```python
from build123d import *

# Parameters (mm, degrees)
F0_R     = 3
F1_DEPTH = 3
F3_DEPTH = 11.5
F4_R     = 0.5
F6_DEPTH = 3.5
F7_D     = 3


with BuildPart() as f1:
    # F0 (on Top) → F1 (new body)
    with BuildSketch(Plane.XY):
        with BuildLine():
            ThreePointArc((-53.0873338103, 3.9548860426), (-48.0828963467, 9.2999784643), (-46.2654588103, 16.393026337))
            ThreePointArc((-46.2654588103, 16.393026337), (-48.0828963467, 23.4860742098), (-53.0873338103, 28.8311666315))
            ThreePointArc((-53.0873338103, 28.8311666315), (-61.0154588103, 31.143026337), (-68.9435838103, 28.8311666315))
            ThreePointArc((-68.9435838103, 28.8311666315), (-75.7654588103, 16.393026337), (-68.9435838103, 3.9548860426))
            ThreePointArc((-68.9435838103, 3.9548860426), (-61.0154588103, 1.643026337), (-53.0873338103, 3.9548860426))
        make_face()
        with BuildLine():
            ThreePointArc((-68.9435838103, 3.9548860426), (-75.7654588103, 16.393026337), (-68.9435838103, 28.8311666315))
            Line((-68.9435838103, 28.8311666315), (-83.1654588103, 19.7660813321))
            ThreePointArc((-83.1654588103, 19.7660813321), (-79.0919204042, 19.9001619204), (-77.0154588103, 16.393026337))
            ThreePointArc((-77.0154588103, 16.393026337), (-79.0919204042, 12.8858907537), (-83.1654588103, 13.0199713419))
            Line((-83.1654588103, 13.0199713419), (-68.9435838103, 3.9548860426))
        make_face()
        with BuildLine():
            ThreePointArc((-53.0873338103, 28.8311666315), (-48.0828963467, 23.4860742098), (-46.2654588103, 16.393026337))
            ThreePointArc((-46.2654588103, 16.393026337), (-48.0828963467, 9.2999784643), (-53.0873338103, 3.9548860426))
            Line((-53.0873338103, 3.9548860426), (-38.8654588103, 13.0199713419))
            ThreePointArc((-38.8654588103, 13.0199713419), (-45.0154588103, 16.393026337), (-38.8654588103, 19.7660813321))
            Line((-38.8654588103, 19.7660813321), (-53.0873338103, 28.8311666315))
        make_face()
        with BuildLine():
            ThreePointArc((-37.0154588103, 16.393026337), (-37.508323227, 18.3165647432), (-38.8654588103, 19.7660813321))
            ThreePointArc((-38.8654588103, 19.7660813321), (-45.0154588103, 16.393026337), (-38.8654588103, 13.0199713419))
            ThreePointArc((-38.8654588103, 13.0199713419), (-37.508323227, 14.4694879309), (-37.0154588103, 16.393026337))
        make_face()
        with Locations((-41.0154588103, 16.393026337)):
            Circle(F0_R, mode=Mode.SUBTRACT)
        with BuildLine():
            ThreePointArc((-77.0154588103, 16.393026337), (-79.0919204042, 19.9001619204), (-83.1654588103, 19.7660813321))
            ThreePointArc((-83.1654588103, 19.7660813321), (-85.0154588103, 16.393026337), (-83.1654588103, 13.0199713419))
            ThreePointArc((-83.1654588103, 13.0199713419), (-79.0919204042, 12.8858907537), (-77.0154588103, 16.393026337))
        make_face()
        with Locations((-81.0154588103, 16.393026337)):
            Circle(F0_R, mode=Mode.SUBTRACT)
    extrude(amount=F1_DEPTH)

    # F2 (on face) → F3 (join)
    with BuildSketch(Plane.XY.offset(3)):
        with BuildLine():
            ThreePointArc((-53.0873338103, 3.9548860426), (-48.0828963467, 9.2999784643), (-46.2654588103, 16.393026337))
            ThreePointArc((-46.2654588103, 16.393026337), (-48.0828963467, 23.4860742098), (-53.0873338103, 28.8311666315))
            ThreePointArc((-53.0873338103, 28.8311666315), (-61.0154588103, 31.143026337), (-68.9435838103, 28.8311666315))
            ThreePointArc((-68.9435838103, 28.8311666315), (-75.7654588103, 16.393026337), (-68.9435838103, 3.9548860426))
            ThreePointArc((-68.9435838103, 3.9548860426), (-61.0154588103, 1.643026337), (-53.0873338103, 3.9548860426))
        make_face()
    extrude(amount=F3_DEPTH)

    # F4
    f4_edges = [f1.edges().sort_by_distance(p)[0] for p in [
        (-53.087334, 28.831167, 14.5),
    ]]
    fillet(f4_edges, radius=F4_R)

    # F0 (on Top) → F6 (join)
    with BuildSketch(Plane.XY):
        with Locations((-41.0154588103, 16.393026337)):
            Circle(F0_R)
        with Locations((-81.0154588103, 16.393026337)):
            Circle(F0_R)
    extrude(amount=F6_DEPTH)

    # F7 (through all)
    with Locations(Plane(origin=(0, 0, 0), x_dir=(1, 0, 0), z_dir=(0, 0, -1))):
        with Locations((-81.0154588103, -16.393026337), (-41.0154588103, -16.393026337)):
            Hole(F7_D / 2)


solid = f1.part
```
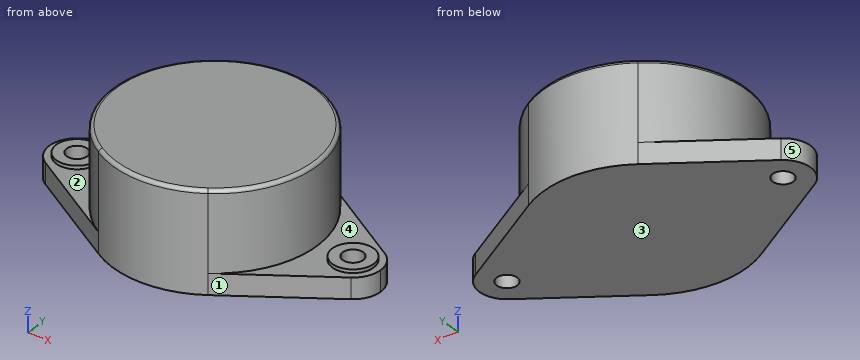
Work out the finished part from the listing and answer in its coordinate system (mm). Face numbers are marked on the shaded views. A direction names the side the tool comes from. Round coordinates to 2 decimals unless told otherwise and drop trailing zeros. Order: outer loops, then holes, each group sorted by start corner. A loop starts at its lowest first (then second) coordinate and runs counter-clockwise, first axis right, second up.
Q1. A cutting plane is placed at C-C, the plane z = 6.5. Determine the outline of the cut face in (x, y).
Solution:
outline: circle Ø29.5 at (-61.02, 16.39)
Q2. A cutting plane is placed at A-A, the plane z = 1.25. Determine the outline of the cut face in (x, y).
Solution:
outline: (-83.17, 13.02) - (-68.94, 3.95) arc R14.75 ccw to (-53.09, 3.95) - (-38.87, 13.02) arc R4 ccw to (-38.87, 19.77) - (-53.09, 28.83) arc R14.75 ccw to (-68.94, 28.83) - (-83.17, 19.77) arc R4 ccw to start; hole circle Ø3 at (-81.02, 16.39); hole circle Ø3 at (-41.02, 16.39)
Q3. Given pin 1 Ø3 at (y, z) = (5, 2.5) entering from +X; pin 2 Ø3 at (x, y) = (-40.5, 15.5) entering from +Z; pin 3 Ø5 at (y, z) = (6, 4.5) entering from -X; pin 4 Ø1.8 at (x, y) = (-41.02, 16.39) entering from -Z, each flat-ended and moving along its own axis, determine where each tip first touches the part or whether it passes through.
Solution:
pin 1: stops at x = -49.09
pin 2: stops at z = 3.5
pin 3: stops at x = -75.29
pin 4: passes through
Q4. A cutting plane is placed at B-B, the plane x = -40.5. Determine the outline of the cut face in (y, z), then the cut area to 3 significant figures.
Solution:
outline: (11.98, 0) - (14.98, 0) - (14.98, 3.5) - (13.44, 3.5) - (13.44, 3) - (11.98, 3) - close; (17.8, 0) - (20.81, 0) - (20.81, 3) - (19.35, 3) - (19.35, 3.5) - (17.8, 3.5) - close
area: 19.6 mm2
Q5. A tool of negligible diameter and unlimited length cuts with its end or side. For the marked faces 4 and 5, from which of +Z, -Z, +X, -X, +Y, -Y can it reach the whole face along a straight path? Write none if from no direction.
Solution:
face 4: +Z
face 5: +Z, -Z, -X
Q6. Find the intervals of material crossed by line 1 along Z through (x, y) = (-49, 24.25); line 2 along Z through (x, y) = (-44, 10.25); line 3 along X through (y, z) = (19, 7.75), in increasing order.
Solution:
line 1: z = 0 to 14.49
line 2: z = 0 to 3
line 3: x = -75.53 to -46.5
Q7. The mould has two halves that part along X. Classify the marked faces 1, 2 and 3: pulls with the +X half, pulls with the -X half, needs draft (parallel to the pull), parting line crosses it, or undercut.
Solution:
face 1: pulls with the +X half
face 2: undercut
face 3: needs draft
